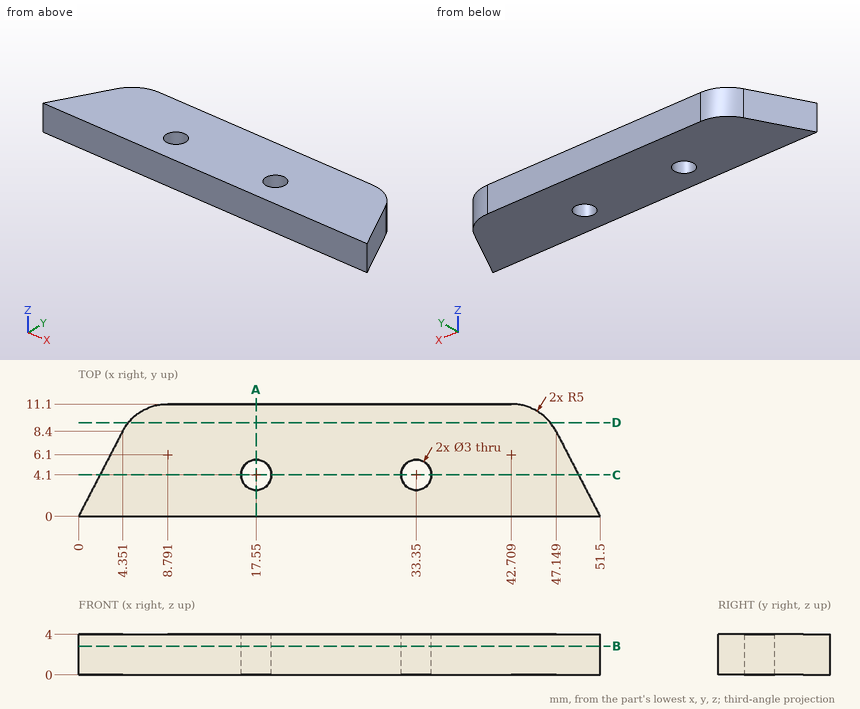
Part print with two shaded views. Sizes in mm from the minimum x, y, z corner. Round coordinates to 2 decimals unless told otherwise and drop trailing zeros. Write each loop counter-clockwise with the first axis right and the second up, starting at its lowest first coordinate (ties: lowest second). Pieces come first, ordered by that corner, then holes. Notation, with made-up numbers: M -16,9 L -9,9 A21 cw -9,44 Z; hole C 10,8 d6. An arc over 180 degrees is marked long. Put each result on its own line as item: value. Start each with the question number.
1) Pin check, flat tips, straight feed: pin 1 Ø2.5 at (x, y) = (33.35, 4.1) entering from -Z; pin 2 Ø1 at (y, z) = (9, 0.5) entering from +X (1 decimal). Stop position of each tip, or through.
2) Drill centre lines: probe 1 along X at (y, z) = (3, 2.05) (1 decimal); probe 2 along X at (y, z) = (4.1, 2.3); probe 3 along Y at (x, z) = (17, 0.8) (1 decimal). Where is each one in solid material? Low to high. Write a range as [from, to].
3) Saw through at B-B, the plane z = 2.85. Write the cut outline in (x, y), and give its area (3 significant figures).
4) Saw through at D-D, the plane y = 9.25. Write the cut outline in (x, z), and give its area (3 significant figures).
5) Saw through at A-A, the plane x = 17.55. Write the cut outline in (y, z), and give its area (3 significant figures).
6) Saw through at C-C, the plane y = 4.1. Write the cut outline in (x, z), and give its area (3 significant figures).
Resolved:
1. pin 1: through
1. pin 2: x = 47.1
2. probe 1: [1.6, 16.5], [18.6, 32.3], [34.4, 49.9]
2. probe 2: [2.12, 16.05], [19.05, 31.85], [34.85, 49.38]
2. probe 3: [0, 2.7], [5.5, 11.1]
3. outline: M 0,0 L 51.5,0 L 47.15,8.4 A5 ccw 42.71,11.1 L 8.79,11.1 A5 ccw 4.35,8.4 Z; hole C 17.55,4.1 d3; hole C 33.35,4.1 d3
3. area: 491 mm²
4. outline: M 4.91,0 L 46.59,0 L 46.59,4 L 4.91,4 Z
4. area: 167 mm²
5. outline: M 0,0 L 2.6,0 L 2.6,4 L 0,4 Z; M 5.6,0 L 11.1,0 L 11.1,4 L 5.6,4 Z
5. area: 32.4 mm²
6. outline: M 2.12,0 L 16.05,0 L 16.05,4 L 2.12,4 Z; M 19.05,0 L 31.85,0 L 31.85,4 L 19.05,4 Z; M 34.85,0 L 49.38,0 L 49.38,4 L 34.85,4 Z
6. area: 165 mm²
